```python
from build123d import *

# Parameters (mm, degrees)
F0_R     = 45
F0_R_2   = 30
F1_DEPTH = 2
F2_R     = 39
F2_R_2   = 36
F3_DEPTH = 2
F4_R     = 0.99999


# Not quite as in the source:
# - a fillet or chamfer is up to 0.001 mm smaller than in the source, because OpenCascade refuses the exact size


with BuildPart() as f1:
    # F0 (on Top) → F1 (new body)
    with BuildSketch(Plane.XY):
        Circle(F0_R)
        Circle(F0_R_2, mode=Mode.SUBTRACT)
    extrude(amount=F1_DEPTH)

    # F2 (on face) → F3 (join)
    with BuildSketch(Plane.XY.offset(2)):
        Circle(F2_R)
        Circle(F2_R_2, mode=Mode.SUBTRACT)
    extrude(amount=F3_DEPTH)

    # F4 (radius 1 in the source; OpenCascade refuses exactly that, so slightly less here)
    f4_edges = [f1.edges().sort_by_distance(p)[0] for p in [
        (-39, 0, 2),
        (-39, 0, 4),
        (-36, 0, 4),
        (-36, 0, 2),
    ]]
    fillet(f4_edges, radius=F4_R)


solid = f1.part
```
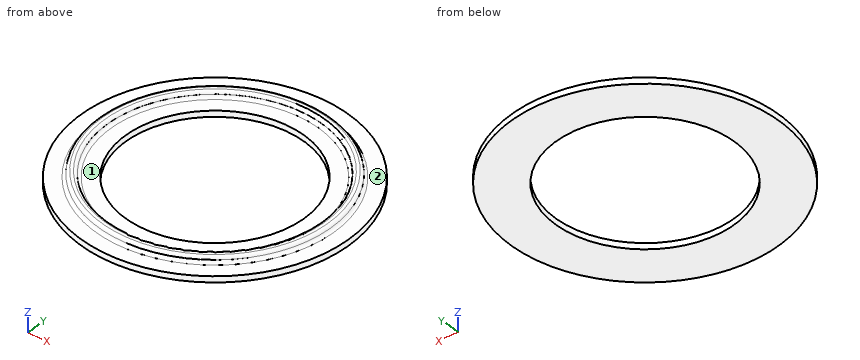
Here's how the part is built. I have some questions about the finished solid (model axes, mm). Face numbers are marked on the shaded views. Give positions to 0.01 mm unless a question says otherwise; leave off trailing zeros. Write each loop counter-clockwise with the first axis right and the second up, starting at its lowest first coordinate (ties: lowest second). Pieces come first, ordered by that corner, then holes.
(1) If I drill on L1, parallel to Y at x = 0, z = 3.05; L2, parallel to Y at x = -23, z = 1.4; L3, parallel to X at y = 24, z = 2.5, over which ranges is the centre line in solid material (lowest first)?
Output values:
L1: y = -39 to -36, 36 to 39
L2: y = -38.68 to -19.26, 19.26 to 38.68
L3: x = -30.91 to -26.65, 26.65 to 30.91
(2) Thinking about a two-plate mould opening in X: for the marked faces 1 and 2, which applies, pulls with the +X half, pulls with the -X half, needs draft (parallel to the pull), parting line crosses it, or undercut?
Output values:
face 1: undercut
face 2: needs draft
(3) Will these pins go through, and if not, where does the flat tip stop? pin 1 (1 mm diameter, centred on y = -1.5, z = 1.5, fed in from -X); pin 2 (2 mm diameter, centred on x = 32, z = 1, fed in from -Y); pin 3 (21 mm diameter, centred on x = 16, y = -13.5, fed in from +Z).
Output values:
pin 1: stops at x = -44.99
pin 2: stops at y = -32.62
pin 3: stops at z = 2
(4) Imagine slicing it at C-C, the plane z = 1.2. Write out the boundary of the cut face in (x, y), and give its area (3 significant figures).
Output values:
outline: circle Ø90 at (0, 0); hole circle Ø60 at (0, 0)
area: 3,530 mm2
